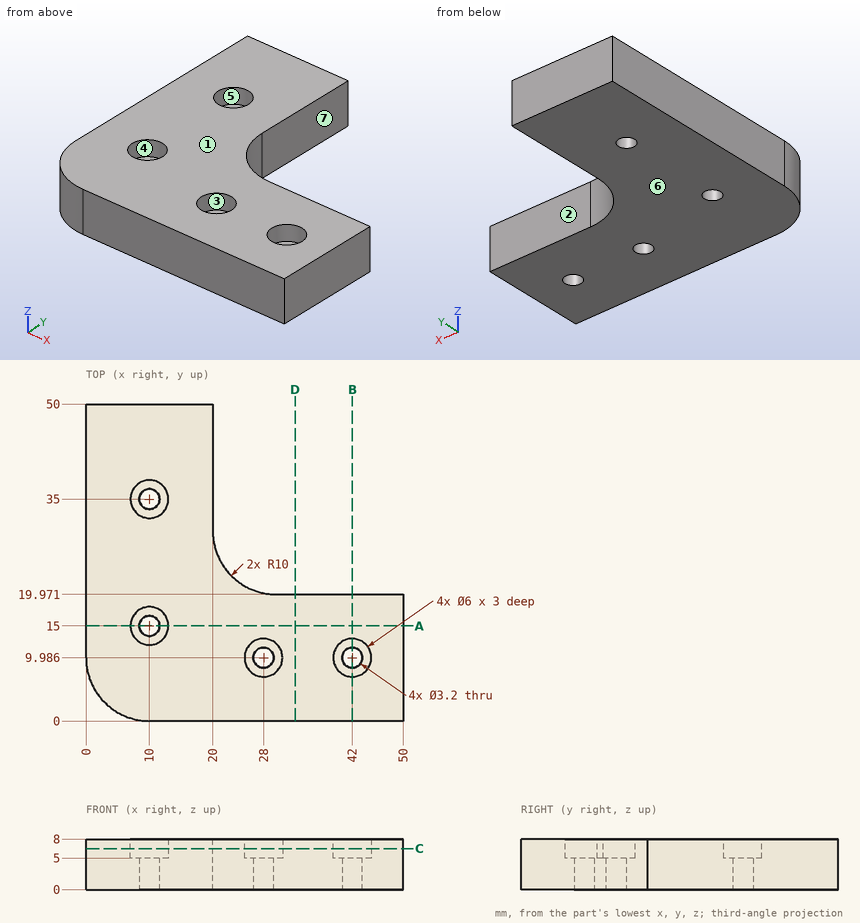
Study the drawing (mm; zero at the part's minimum x, y, z) and answer. A direction names the side the tool comes from. Round coordinates to 2 decimals unless told otherwise and drop trailing zeros. Loops run counter-clockwise (first coordinate to the right, second up) from the corner with the lowest first, then second, coordinate; pieces in that order, holes last.
Q1. For a pull along Y with two mould halves and no side action, classify the marked faces 1, 2, 3 and 4 as released by +Y, released by -Y, zero draft, split by the parting line, or undercut.
Q2. Section B-B, the plane x = 42 is taken. Determine the outline of the cut face in (y, z) (1 decimal), then the cut area to 3 significant figures.
Q3. Which of the six approach directions +Z, -Z, +X, -X, +Y, -Y give full straight-line access (tool end or side, diameter ignored) to the marked faces 5, 6 and 7?
Q4. Section A-A, the plane y = 15 is taken. Determine the outline of the cut face in (x, z), then the cut area to 3 significant figures.
Q5. Given pin 1 Ø4 at (x, z) = (35.5, 6) entering from +Y; pin 2 Ø4 at (x, y) = (42, 9.99) entering from +Z; pin 3 Ø1.9 at (x, y) = (10, 15) entering from -Z; pin 4 Ø4 at (y, z) = (41, 2.5) entering from +X, each flat-ended and moving along its own axis, determine where each tip first touches the part or whether it passes through.
Q6. Section C-C, the plane z = 6.5 is taken. Determine the outline of the cut face in (x, y) (1 decimal), then the cut area to 3 significant figures.
Q7. Find the intervals of material crossed by line 1 (Y direction, x = 10, z = 6.7); line 2 (Y direction, x = 10, z = 1.1); line 3 (X direction, y = 12.5, z = 5.75) (1 decimal), in increasing order.
Q8. Section D-D, the plane x = 33 is taken. Determine the outline of the cut face in (y, z), then the cut area to 3 significant figures.
Completed:
1. face 1: zero draft
1. face 2: released by +Y
1. face 3: undercut
1. face 4: undercut
2. outline: (0, 0) - (8.4, 0) - (8.4, 5) - (7, 5) - (7, 8) - (0, 8) - close; (11.6, 0) - (20, 0) - (20, 8) - (13, 8) - (13, 5) - (11.6, 5) - close
2. area: 126 mm2
3. face 5: +Z
3. face 6: -Z, +X, -X, +Y, -Y
3. face 7: +Z, -Z, +X, +Y
4. outline: (0, 0) - (8.4, 0) - (8.4, 5) - (7, 5) - (7, 8) - (0, 8) - close; (11.6, 0) - (50, 0) - (50, 8) - (13, 8) - (13, 5) - (11.6, 5) - close
4. area: 366 mm2
5. pin 1: stops at y = 19.97
5. pin 2: stops at z = 5
5. pin 3: passes through
5. pin 4: stops at x = 20
6. outline: (0, 10) arc R10 ccw to (10, 0) - (50, 0) - (50, 20) - (30, 20) arc R10 cw to (20, 30) - (20, 50) - (0, 50) - close; hole circle Ø6 at (10, 15); hole circle Ø6 at (10, 35); hole circle Ø6 at (28, 10); hole circle Ø6 at (42, 10)
6. area: 1,490 mm2
7. line 1: y = 0 to 12, 18 to 32, 38 to 50
7. line 2: y = 0 to 13.4, 16.6 to 33.4, 36.6 to 50
7. line 3: x = 0 to 8.3, 11.7 to 26.4, 29.6 to 40.4, 43.6 to 50
8. outline: (0, 0) - (19.97, 0) - (19.97, 8) - (0, 8) - close
8. area: 160 mm2
